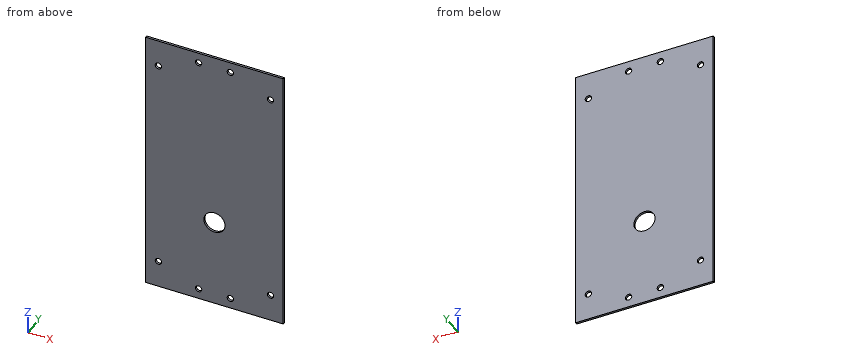
from build123d import *

# Parameters (mm, degrees)
SKETCH_1_W          = 65
SKETCH_1_H          = 128
SKETCH_1_R          = 1.5
EXTRUDE_1_DEPTH     = 1
SKETCH_2_R          = 1.5
CUT_EXTRUDE_1_DEPTH = 2
SKETCH_3_R          = 5
CUT_EXTRUDE_2_DEPTH = 10


with BuildPart() as part:
    # Эскиз1 → Бобышка-Вытянуть1 (new body)
    with BuildSketch(Plane(origin=(0, 0, 0), x_dir=(1, 0, 0), z_dir=(0, 1, 0))):
        with Locations((-41.85845893, -10.35845893)):
            Rectangle(SKETCH_1_W, SKETCH_1_H)
        with Locations((-68.35845893, 40.64154107)):
            Circle(SKETCH_1_R, mode=Mode.SUBTRACT)
        with Locations((-15.35845893, 40.64154107)):
            Circle(SKETCH_1_R, mode=Mode.SUBTRACT)
        with Locations((-15.35845893, -61.35845893)):
            Circle(SKETCH_1_R, mode=Mode.SUBTRACT)
        with Locations((-68.35845893, -61.35845893)):
            Circle(SKETCH_1_R, mode=Mode.SUBTRACT)
    extrude(amount=EXTRUDE_1_DEPTH)

    # Эскиз2 → Вырез-Вытянуть1 (cut, through all)
    with BuildSketch(Plane(origin=(0, 1, 0), x_dir=(1, 0, 0), z_dir=(0, 1, 0))):
        with Locations((-49.35845893, 48.64154107)):
            Circle(SKETCH_2_R)
        with Locations((-34.35845893, 48.64154107)):
            Circle(SKETCH_2_R)
        with Locations((-34.35845893, -69.35845893)):
            Circle(SKETCH_2_R)
        with Locations((-49.35845893, -69.35845893)):
            Circle(SKETCH_2_R)
    extrude(amount=-CUT_EXTRUDE_1_DEPTH, mode=Mode.SUBTRACT)

    # Эскиз3 → Вырез-Вытянуть2 (cut)
    with BuildSketch(Plane(origin=(0, 1, 0), x_dir=(1, 0, 0), z_dir=(0, 1, 0))):
        with Locations((-41.85845893, 11.48154107)):
            Circle(SKETCH_3_R)
    extrude(amount=-CUT_EXTRUDE_2_DEPTH, mode=Mode.SUBTRACT)


solid = part.part
Verification items for the finished model (mm, model axes). Coordinates: 2 decimals unless noted, no trailing zeros. Order: outer loops, then holes, each group sorted by start corner. A loop starts at its lowest first (then second) coordinate and runs counter-clockwise, first axis right, second up. Notation, with made-up numbers: (-9.75, 3.5) -> (48.25, 3.5) arc R18 cw to (48.25, 21.5) -> close; hole circle Ø3 at (3, 76). An arc over 180 degrees is marked (long way). Use CSV: the item, a comma, the result in double quotes. Start each with the question number.
Q1. Thickness scan on line 1 along Z through (x, y) = (-14, 0.15); line 2 along X through (y, z) = (0.5, -12.5); line 3 along X through (y, z) = (0.15, -15). Record the ranges inside material, lowest first.
Q2. Section check C-C, the plane z = -8. Record the cut outline in (x, y).
Q3. Depth check by flat-ended pin: P1, Ø2.5, axis at x = -15.36, z = -40.64, coming from the +Y side. Enter the tip coordinate at first touch or a pass-through.
Q4. Section check D-D, the plane y = 0.7. Give the number of separate pieces and of enclosed holes in the cut face, and give its area (3 significant figures).
Q5. Section check B-B, the plane x = -15.5. Record the cut outline in (y, z), and give its area (3 significant figures).
Q6. Section check A-A, the plane x = -42. Record the cut outline in (y, z).
Returned:
1,line 1,"z = -53.64 to -41.28, -40.01 to 60.72, 61.99 to 74.36"
1,line 2,"x = -74.36 to -46.75, -36.96 to -9.36"
1,line 3,"x = -74.36 to -45.41, -38.31 to -9.36"
2,outline,"(-74.36, 0) -> (-45.45, 0) -> (-45.45, 1) -> (-74.36, 1) -> close; (-38.27, 0) -> (-9.36, 0) -> (-9.36, 1) -> (-38.27, 1) -> close"
3,P1,"passes through"
4,separate pieces,"1"
4,enclosed holes,"9"
4,area,"8,180 mm^2"
5,outline,"(0, -53.64) -> (1, -53.64) -> (1, -42.13) -> (0, -42.13) -> close; (0, -39.15) -> (1, -39.15) -> (1, 59.87) -> (0, 59.87) -> close; (0, 62.85) -> (1, 62.85) -> (1, 74.36) -> (0, 74.36) -> close"
5,area,"122 mm^2"
6,outline,"(0, -53.64) -> (1, -53.64) -> (1, -16.48) -> (0, -16.48) -> close; (0, -6.48) -> (1, -6.48) -> (1, 74.36) -> (0, 74.36) -> close"
